The listing builds one solid part. Answer for the finished solid, in the listing's coordinates (mm). Face numbers are marked on the shaded views. Round coordinates to 2 decimals unless told otherwise and drop trailing zeros. Write each loop counter-clockwise with the first axis right and the second up, starting at its lowest first coordinate (ties: lowest second). Pieces come first, ordered by that corner, then holes.
Item 1: Find section A-A on z = 0. Give the vertices of the cut face in (x, y).
Item 2: Find section D-D on x = 43.5. Give the vertices of the cut face in (y, z), then the cut area to 3 significant figures.
Item 3: Each of these flat-tipped pins is pushed along its axis until it touches: pin 1 (8 mm diameter, centred on x = -22, y = 7.5, fed in from +Z); pin 2 (2.5 mm diameter, centred on x = -4, z = 12, fed in from +Y); pin 3 (1 mm diameter, centred on x = 26.5, y = 7, fed in from -Z). Where does it stop, or does it pass through?
Item 4: Find section B-B on y = 6.25. Give the vertices of the cut face in (x, z), then the cut area to 3 significant figures.
Item 5: For a pull along Z with two mould halves and no side action, classify the marked faces 1, 2 and 3 as +Z half, -Z half, draft (parallel to the pull), parting line (faces both ways), or undercut.
Item 6: Find section C-C on z = 50. Give the vertices of the cut face in (x, y), then the cut area to 3 significant figures.
Item 7: Find the intervals of material crossed by probe 1 along X at (y, z) = (6.5, 0); probe 2 along X at (y, z) = (7, -7.5); probe 3 along X at (y, z) = (15.25, 11.5), in increasing order.
```python
from build123d import *

# Parameters (mm, degrees)
SKETCH1_R           = 62.5
BOSS_EXTRUDE1_DEPTH = 24
SKETCH2_R           = 10
CUT_EXTRUDE1_DEPTH  = 92.588754768
SKETCH3_R           = 2.384291232
CUT_EXTRUDE2_DEPTH  = 23.873555
CIRPATTERN1_START   = 0.126444925
CIRPATTERN1_DEPTH   = 23.873555075


# Read off the part's stored shape, not the designer's step: CirPattern1
with BuildPart() as part:
    # Sketch1 → Boss-Extrude1 (new body)
    with BuildSketch(Plane(origin=(0, 0, 0), x_dir=(1, 0, 0), z_dir=(0, 1, 0))):
        with Locations(Location((0, 0, 0), (0, 0, 270))):
            Circle(SKETCH1_R)
    extrude(amount=BOSS_EXTRUDE1_DEPTH)

    # Sketch2 → Cut-Extrude1 (cut, through all)
    with BuildSketch(Plane(origin=(0, 0, 0), x_dir=(1, 0, 0), z_dir=(0, 1, 0))):
        with Locations(Location((0, 0, 0), (0, 0, 270))):
            Circle(SKETCH2_R)
    extrude(amount=CUT_EXTRUDE1_DEPTH, mode=Mode.SUBTRACT)

    # Sketch3 → Cut-Extrude2 (cut)
    with BuildSketch(Plane(origin=(0, 24, 0), x_dir=(1, 0, 0), z_dir=(0, 1, 0))):
        with Locations((-11.723740212, 0)):
            Circle(SKETCH3_R)
    extrude(amount=-CUT_EXTRUDE2_DEPTH, mode=Mode.SUBTRACT)

    # CirPattern1 outline → CirPattern1 (cut)
    with BuildSketch(Plane(origin=(0, 0, 0), x_dir=(1, 0, 0), z_dir=(0, 1, 0)).offset(CIRPATTERN1_START)):
        with BuildLine():
            ThreePointArc((-1.611683994, -9.869269208), (-3.090169944, -9.510565163), (-4.497131151, -8.931730594))
            ThreePointArc((-4.497131151, -8.931730594), (-4.359621474, -13.417535237), (-1.611683994, -9.869269208))
        make_face()
        with BuildLine():
            ThreePointArc((-1.611683994, 9.869269208), (-4.359621474, 13.417535237), (-4.497131151, 8.931730594))
            ThreePointArc((-4.497131151, 8.931730594), (-3.090169944, 9.510565163), (-1.611683994, 9.869269208))
        make_face()
        with BuildLine():
            ThreePointArc((8.888195048, -4.582574472), (8.090169944, -5.877852523), (7.104890632, -7.037082429))
            ThreePointArc((7.104890632, -7.037082429), (11.413637196, -8.292492822), (8.888195048, -4.582574472))
        make_face()
        with BuildLine():
            ThreePointArc((8.888195048, 4.582574472), (11.413637196, 8.292492822), (7.104890632, 7.037082429))
            ThreePointArc((7.104890632, 7.037082429), (8.090169944, 5.877852523), (8.888195048, 4.582574472))
        make_face()
    extrude(amount=CIRPATTERN1_DEPTH, mode=Mode.SUBTRACT)


solid = part.part
```
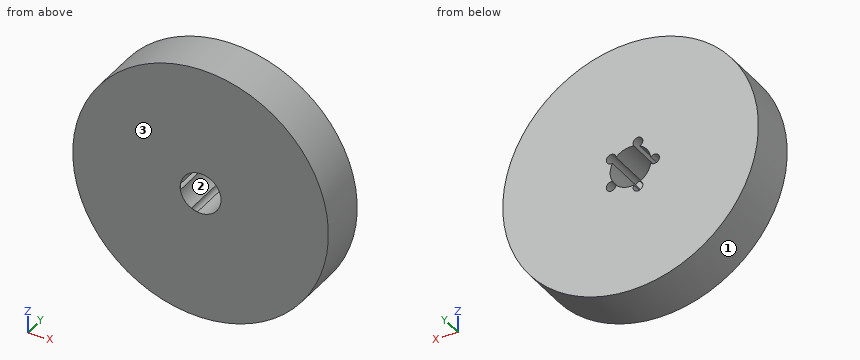
Check values:
1. outline: (-62.5, 0) - (-10, 0) - (-10, 0.13) - (-14.11, 0.13) - (-14.11, 24) - (-62.5, 24) - close; (10, 0) - (62.5, 0) - (62.5, 24) - (10, 24) - close
2. outline: (0, -44.88) - (24, -44.88) - (24, 44.88) - (0, 44.88) - close
2. area: 2,150 mm2
3. pin 1: stops at z = 59.85
3. pin 2: stops at y = 0.13
3. pin 3: stops at z = -56.84
4. outline: circle Ø125 at (0, 0); hole (-9.88, -1.52) arc R10 ccw to (-4.5, -8.93) arc R2.38 ccw (long way) to (-1.61, -9.87) arc R10 ccw to (7.1, -7.04) arc R2.38 ccw (long way) to (8.89, -4.58) arc R10 ccw to (8.89, 4.58) arc R2.38 ccw (long way) to (7.1, 7.04) arc R10 ccw to (-1.61, 9.87) arc R2.38 ccw (long way) to (-4.5, 8.93) arc R10 ccw to (-9.88, 1.52) arc R2.38 ccw (long way) to start
4. area: 11,900 mm2
5. face 1: parting line
5. face 2: undercut
5. face 3: draft
6. outline: (-37.5, 0) - (37.5, 0) - (37.5, 24) - (-37.5, 24) - close
6. area: 1,800 mm2
7. probe 1: x = -62.5 to -14.11, 10 to 62.5
7. probe 2: x = -62.05 to -6.61, 6.61 to 7.18, 11.79 to 62.05
7. probe 3: x = -61.43 to -5.98, -1.26 to 61.43
